Verification items for the finished model (mm, model axes). A direction names the side the tool comes from. Give positions to 0.01 mm unless a question says otherwise; leave off trailing zeros. Loops run counter-clockwise (first coordinate to the right, second up) from the corner with the lowest first, then second, coordinate; pieces in that order, holes last. Notation, with made-up numbers: M -13.75,85.25 L 20.25,85.25 A25 ccw 20.25,111.25 Z; hole C 64.25,54 d5. An arc over 180 degrees is marked long. Answer in a Markdown table with one row per item.
```python
from build123d import *

# Parameters (mm, degrees)
SKETCH_1_R        = 110
SKETCH_1_R_2      = 3
SKETCH_1_R_3      = 90
EXTRUDE_1_DEPTH   = 10
SKETCH_1_R_4      = 80
SKETCH_1_R_5      = 75
EXTRUDE_1_2_DEPTH = 10
SKETCH_1_3_R      = 90
SKETCH_1_3_R_2    = 80
SKETCH_1_3_R_3    = 75
EXTRUDE_2_DEPTH   = 5


with BuildPart() as part:
    # Sketch 1 → Extrude 1 (new body)
    with BuildSketch(Plane(origin=(0, 0, 0), x_dir=(1, 0, 0), z_dir=(0, 1, 0))):
        with Locations(Location((0, 0, 0), (0, 0, 270))):
            Circle(SKETCH_1_R)
        with Locations(Location((-38.268343237, 92.387953251, 0), (0, 0, 270))):
            Circle(SKETCH_1_R_2, mode=Mode.SUBTRACT)
        with Locations(Location((-70.710678119, 70.710678119, 0), (0, 0, 270))):
            Circle(SKETCH_1_R_2, mode=Mode.SUBTRACT)
        with Locations(Location((-92.387953251, 38.268343237, 0), (0, 0, 270))):
            Circle(SKETCH_1_R_2, mode=Mode.SUBTRACT)
        with Locations(Location((-100, 0, 0), (0, 0, 270))):
            Circle(SKETCH_1_R_2, mode=Mode.SUBTRACT)
        with Locations(Location((-92.387953251, -38.268343237, 0), (0, 0, 270))):
            Circle(SKETCH_1_R_2, mode=Mode.SUBTRACT)
        with Locations(Location((-70.710678119, -70.710678119, 0), (0, 0, 270))):
            Circle(SKETCH_1_R_2, mode=Mode.SUBTRACT)
        with Locations(Location((-38.268343237, -92.387953251, 0), (0, 0, 270))):
            Circle(SKETCH_1_R_2, mode=Mode.SUBTRACT)
        with Locations(Location((0, -100, 0), (0, 0, 270))):
            Circle(SKETCH_1_R_2, mode=Mode.SUBTRACT)
        with Locations(Location((38.268343237, -92.387953251, 0), (0, 0, 270))):
            Circle(SKETCH_1_R_2, mode=Mode.SUBTRACT)
        with Locations(Location((70.710678119, -70.710678119, 0), (0, 0, 270))):
            Circle(SKETCH_1_R_2, mode=Mode.SUBTRACT)
        with Locations(Location((92.387953251, -38.268343237, 0), (0, 0, 270))):
            Circle(SKETCH_1_R_2, mode=Mode.SUBTRACT)
        with Locations(Location((100, 0, 0), (0, 0, 270))):
            Circle(SKETCH_1_R_2, mode=Mode.SUBTRACT)
        with Locations(Location((92.387953251, 38.268343237, 0), (0, 0, 270))):
            Circle(SKETCH_1_R_2, mode=Mode.SUBTRACT)
        with Locations(Location((70.710678119, 70.710678119, 0), (0, 0, 270))):
            Circle(SKETCH_1_R_2, mode=Mode.SUBTRACT)
        with Locations(Location((38.268343237, 92.387953251, 0), (0, 0, 270))):
            Circle(SKETCH_1_R_2, mode=Mode.SUBTRACT)
        with Locations(Location((0, 100, 0), (0, 0, 270))):
            Circle(SKETCH_1_R_2, mode=Mode.SUBTRACT)
        with Locations(Location((0, 0, 0), (0, 0, 270))):
            Circle(SKETCH_1_R_3, mode=Mode.SUBTRACT)
    extrude(amount=EXTRUDE_1_DEPTH)



with BuildPart() as body_2:
    # Sketch 1 → Extrude 1 2 (new body)
    with BuildSketch(Plane(origin=(0, 0, 0), x_dir=(1, 0, 0), z_dir=(0, 1, 0))):
        with Locations(Location((0, 0, 0), (0, 0, 270))):
            Circle(SKETCH_1_R_4)
        with Locations(Location((0, 0, 0), (0, 0, 270))):
            Circle(SKETCH_1_R_5, mode=Mode.SUBTRACT)
    extrude(amount=EXTRUDE_1_2_DEPTH)


with BuildPart() as part_1:
    add(part.part)

    add(body_2.part)  # Extrude 2 merges body 2
    # Sketch 1_3 → Extrude 2 (add)
    # profile 1 of 2: a face of its own
    with BuildSketch(Plane(origin=(0, 0, 0), x_dir=(1, 0, 0), z_dir=(0, 1, 0))):
        with Locations(Location((0, 0, 0), (0, 0, 270))):
            Circle(SKETCH_1_3_R)
        with Locations(Location((0, 0, 0), (0, 0, 270))):
            Circle(SKETCH_1_3_R_2, mode=Mode.SUBTRACT)
    # profile 2 of 2: a face of its own
    with BuildSketch(Plane(origin=(0, 0, 0), x_dir=(1, 0, 0), z_dir=(0, 1, 0))):
        with Locations(Location((0, 0, 0), (0, 0, 270))):
            Circle(SKETCH_1_3_R_3)
    extrude(amount=EXTRUDE_2_DEPTH)


solid = part_1.part
```
Item 1: Scan lines: L1, parallel to X at y = 7.5, z = -35; L2, parallel to Z at x = 8, y = 7.75; L3, parallel to X at y = 7, z = 25.5. Record each from-to range of solid material in increasing order. Write a range as [from, to].
Reported:
| item | result |
|---|---|
| L1 | x = [-104.28, -82.92], [-71.94, -66.33], [66.33, 71.94], [82.92, 104.28] |
| L2 | z = [-109.71, -89.64], [-79.6, -74.57], [74.57, 79.6], [89.64, 109.71] |
| L3 | x = [-107, -86.31], [-75.83, -70.53], [70.53, 75.83], [86.31, 107] |
Item 2: Release check for a two-part mould opening along X. For faces 3 (the cylindrical face through (-97.59, 4.93, 50.76)), 4 (the cylindrical face through (-38.136, 4.93, -95.385)), 5 (the flat face through (71.5, 10, 23.3)), 6 (the flat face through (-52.9, 5, -60.4)) record: released by +X, released by -X, zero draft, split by the parting line, or undercut.
Reported:
| item | result |
|---|---|
| face 3 | split by the parting line |
| face 4 | undercut |
| face 5 | zero draft |
| face 6 | undercut |
Item 3: Sectioned sample at B-B (x = 0). Record the cut outline in (y, z), and give its area (3 significant figures).
Reported:
| item | result |
|---|---|
| outline | M 0,-110 L 10,-110 L 10,-103 L 0,-103 Z; M 0,-97 L 10,-97 L 10,-90 L 5,-90 L 5,-80 L 10,-80 L 10,-75 L 5,-75 L 5,75 L 10,75 L 10,80 L 5,80 L 5,90 L 10,90 L 10,97 L 0,97 Z; M 0,103 L 10,103 L 10,110 L 0,110 Z |
| area | 1,230 mm^2 |
Item 4: Tool access check on faces 1 (the cylindrical face through (-45.636, 7.465, -59.517)), 2 (the cylindrical face through (38.4, 4.93, -95.385)). Record the directions out of +Z, -Z, +X, -X, +Y, -Y that give a thin tool (end or side, any length) a straight path to the whole face; none if there is none.
Reported:
| item | result |
|---|---|
| face 1 | +Y |
| face 2 | +Y, -Y |
Item 5: Sectioned sample at C-C (y = 2.25). State how many separate pieces and enclosed holes the cut face has, and give its area (3 significant figures).
Reported:
| item | result |
|---|---|
| separate pieces | 1 |
| enclosed holes | 16 |
| area | 37,600 mm^2 |
Item 6: Go/stop test with flat-tipped pins: pin 1 (3 mm diameter, centred on y = 3, z = -53, fed in from -X); pin 2 (1 mm diameter, centred on y = 2, z = 54, fed in from +X); pin 3 (6 mm diameter, centred on x = 27, y = 8, fed in from +Z). Record where each tip stops, or that it passes through.
Reported:
| item | result |
|---|---|
| pin 1 | stops at x = -97.2 |
| pin 2 | stops at x = 96.11 |
| pin 3 | stops at z = 107.35 |
Item 7: Sectioned sample at D-D (z = -100). Record the cut outline in (x, y), and give its area (3 significant figures).
Reported:
| item | result |
|---|---|
| outline | M -45.83,0 L -3,0 L -3,10 L -45.83,10 Z; M 3,0 L 45.83,0 L 45.83,10 L 3,10 Z |
| area | 857 mm^2 |
Item 8: Sectioned sample at A-A (z = 0). Record the cut outline in (x, y), and give its area (3 significant figures).
Reported:
| item | result |
|---|---|
| outline | M -110,0 L -103,0 L -103,10 L -110,10 Z; M -97,0 L 97,0 L 97,10 L 90,10 L 90,5 L 80,5 L 80,10 L 75,10 L 75,5 L -75,5 L -75,10 L -80,10 L -80,5 L -90,5 L -90,10 L -97,10 Z; M 103,0 L 110,0 L 110,10 L 103,10 Z |
| area | 1,230 mm^2 |
